Here's how the part is built. I have some questions about the finished solid (model axes, mm). Face numbers are marked on the shaded views. A direction names the side the tool comes from. Round coordinates to 2 decimals unless told otherwise and drop trailing zeros. Order: outer loops, then holes, each group sorted by start corner. A loop starts at its lowest first (then second) coordinate and runs counter-clockwise, first axis right, second up. Notation, with made-up numbers: M -6,-37 L 21,-37 A15 cw 21,-20 Z; hole C 7,-0.75 d4. An arc over 180 degrees is marked long. Use one line per item in the form item = value. Start each with the question number.
```python
from build123d import *
from OCP.BRepFilletAPI import BRepFilletAPI_MakeChamfer

# Parameters (mm, degrees)
SKETCH_1_W               = 126.5
SKETCH_1_H               = 82.5
SKETCH_1_W_2             = 28
SKETCH_1_H_2             = 28
EXTRUDE_1_DEPTH          = 8
SKETCH_2_W               = 126.5
SKETCH_2_H               = 23.75
EXTRUDE_2_DEPTH          = 0.25
CHAMFER_1_SIZE           = 1
CHAMFER_1_SIZE2          = 11.430052303
FILLET_1_R               = 2
FILLET_2_R               = 1
CUT_EXTRUDE_1_DEPTH      = 76.935005103
CUT_EXTRUDE_1_DEPTH_BACK = 76.935005103
SKETCH_3_R               = 2.1
CHAMFER_2_SIZE           = 6
CHAMFER_2_SIZE2          = 3.464101615
CHAMFER_3_SIZE           = 6
CHAMFER_3_SIZE2          = 3.464101615


with BuildPart() as part:
    # Эскиз1 → Бобышка-Вытянуть1 (new body)
    with BuildSketch(Plane(origin=(0, 0, 0), x_dir=(1, 0, 0), z_dir=(0, 1, 0))):
        Rectangle(SKETCH_1_W, SKETCH_1_H)
        Rectangle(SKETCH_1_W_2, SKETCH_1_H_2, mode=Mode.SUBTRACT)
    extrude(amount=EXTRUDE_1_DEPTH)

    # Эскиз2 → Бобышка-Вытянуть2 (add)
    with BuildSketch(Plane(origin=(0, 8, 0), x_dir=(1, 0, 0), z_dir=(0, 1, 0))):
        with Locations((0, 29.375)):
            Rectangle(SKETCH_2_W, SKETCH_2_H)
        with Locations((0, -29.375)):
            Rectangle(SKETCH_2_W, SKETCH_2_H)
    extrude(amount=EXTRUDE_2_DEPTH)

    # Фаска1: one chamfer whose edges measure the first distance from different faces: ONE call of the kernel's chamfer builder (chamfer() names one face for all edges)
    chamfer_1_edges_1 = [part.edges().sort_by_distance(p)[0] for p in [
        (-63.25, 8, 0),
    ]]
    chamfer_1_side_1 = [part.faces().sort_by_distance(p)[0] for p in [
        (-63.25, 4.072906977, 0),
    ]]
    chamfer_1_edges_2 = [part.edges().sort_by_distance(p)[0] for p in [
        (63.25, 8, 0),
    ]]
    chamfer_1_side_2 = [part.faces().sort_by_distance(p)[0] for p in [
        (63.25, 4.072906977, 0),
    ]]
    chamfer_1 = BRepFilletAPI_MakeChamfer(part.part.solid().wrapped)
    for e in chamfer_1_edges_1:
        chamfer_1.Add(CHAMFER_1_SIZE, CHAMFER_1_SIZE2, e.wrapped, chamfer_1_side_1[0].wrapped)  # the first distance lies on this face
    for e in chamfer_1_edges_2:
        chamfer_1.Add(CHAMFER_1_SIZE, CHAMFER_1_SIZE2, e.wrapped, chamfer_1_side_2[0].wrapped)  # the first distance lies on this face
    add(Compound.cast(chamfer_1.Shape()), mode=Mode.REPLACE)

    # Скругление1
    fillet_1_edges = [part.edges().sort_by_distance(p)[0] for p in [
        (63.25, 7, 0),
        (-63.25, 7, 0),
    ]]
    fillet(fillet_1_edges, radius=FILLET_1_R)

    # Скругление2
    fillet_2_edges = [part.edges().sort_by_distance(p)[0] for p in [
        (-14, 8, 0),
        (14, 8, 0),
    ]]
    fillet(fillet_2_edges, radius=FILLET_2_R)

    # Эскиз3 → Вырез-Вытянуть1 (cut, two sides: drawn at the far end of the back side and taken through both)
    with BuildSketch(Plane(origin=(0, 8, 0), x_dir=(1, 0, 0), z_dir=(0, 1, 0)).offset(-CUT_EXTRUDE_1_DEPTH_BACK)):
        with Locations(Location((-40, 30, 0), (0, 0, 270))):
            Circle(SKETCH_3_R)
        with Locations(Location((40, 30, 0), (0, 0, 270))):
            Circle(SKETCH_3_R)
        with Locations(Location((-40, -30, 0), (0, 0, 270))):
            Circle(SKETCH_3_R)
        with Locations(Location((40, -30, 0), (0, 0, 270))):
            Circle(SKETCH_3_R)
    extrude(amount=CUT_EXTRUDE_1_DEPTH + CUT_EXTRUDE_1_DEPTH_BACK, mode=Mode.SUBTRACT)

    # Фаска2: one chamfer whose edges measure the first distance from different faces: ONE call of the kernel's chamfer builder (chamfer() names one face for all edges)
    chamfer_2_edges_1 = [part.edges().sort_by_distance(p)[0] for p in [
        (-14, 0, 0),
    ]]
    chamfer_2_side_1 = [part.faces().sort_by_distance(p)[0] for p in [
        (-14, 3.5, 0),
    ]]
    chamfer_2_edges_2 = [part.edges().sort_by_distance(p)[0] for p in [
        (14, 0, 0),
    ]]
    chamfer_2_side_2 = [part.faces().sort_by_distance(p)[0] for p in [
        (14, 3.5, 0),
    ]]
    chamfer_2 = BRepFilletAPI_MakeChamfer(part.part.solid().wrapped)
    for e in chamfer_2_edges_1:
        chamfer_2.Add(CHAMFER_2_SIZE, CHAMFER_2_SIZE2, e.wrapped, chamfer_2_side_1[0].wrapped)  # the first distance lies on this face
    for e in chamfer_2_edges_2:
        chamfer_2.Add(CHAMFER_2_SIZE, CHAMFER_2_SIZE2, e.wrapped, chamfer_2_side_2[0].wrapped)  # the first distance lies on this face
    add(Compound.cast(chamfer_2.Shape()), mode=Mode.REPLACE)

    # Фаска3: one chamfer whose edges measure the first distance from different faces: ONE call of the kernel's chamfer builder (chamfer() names one face for all edges)
    chamfer_3_edges_1 = [part.edges().sort_by_distance(p)[0] for p in [
        (0, 0, 14),
    ]]
    chamfer_3_side_1 = [part.faces().sort_by_distance(p)[0] for p in [
        (0, 3.837087991, 14),
    ]]
    chamfer_3_edges_2 = [part.edges().sort_by_distance(p)[0] for p in [
        (0, 0, -14),
    ]]
    chamfer_3_side_2 = [part.faces().sort_by_distance(p)[0] for p in [
        (0, 3.837087991, -14),
    ]]
    chamfer_3 = BRepFilletAPI_MakeChamfer(part.part.solid().wrapped)
    for e in chamfer_3_edges_1:
        chamfer_3.Add(CHAMFER_3_SIZE, CHAMFER_3_SIZE2, e.wrapped, chamfer_3_side_1[0].wrapped)  # the first distance lies on this face
    for e in chamfer_3_edges_2:
        chamfer_3.Add(CHAMFER_3_SIZE, CHAMFER_3_SIZE2, e.wrapped, chamfer_3_side_2[0].wrapped)  # the first distance lies on this face
    add(Compound.cast(chamfer_3.Shape()), mode=Mode.REPLACE)


solid = part.part
```
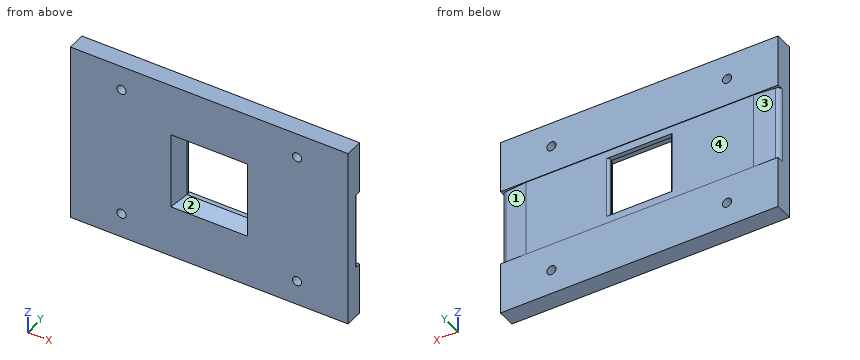
1) If we section it at D-D on z = -30: Write out the boundary of the cut face in (x, y), then the cut area to 3 significant figures.
2) If I drill on line 1 (Z direction, x = -40, y = 3); line 2 (X direction, y = 3, z = -30); line 3 (Z direction, x = -2, y = 6.25), over which ranges is the centre line in solid material (lowest first)?
3) If we section it at A-A on x = 40: Write out the boundary of the cut face in (y, z), then the cut area to 3 significant figures.
4) If we section it at B-B on z = -8: Write out the boundary of the cut face in (x, y), then the cut area to 3 significant figures.
5) If we section it at C-C on x = -7: Write out the boundary of the cut face in (y, z).
6) On a 3-axis mill with a long thin cutter (end or side, diameter ignored), from which of +Z, -Z, +X, -X, +Y, -Y can I reach the whole of each face in a straight line? I mean the marked faces 1, 2, 3 and 4. Say none if no direction works.
7) Will these pins go through, and if not, where does the flat tip stop? pin 1 Ø0.5 at (y, z) = (6.5, -1.5) entering from -X; pin 2 Ø5.5 at (x, z) = (40, 30) entering from -Y; pin 3 Ø1.5 at (x, z) = (50, -2.5) entering from +Y; pin 4 Ø4 at (x, z) = (40, -30) entering from +Y.
Completed:
q1.outline = M -63.25,0 L -42.1,0 L -42.1,8.25 L -63.25,8.25 Z; M -37.9,0 L 37.9,0 L 37.9,8.25 L -37.9,8.25 Z; M 42.1,0 L 63.25,0 L 63.25,8.25 L 42.1,8.25 Z
q1.area = 974 mm²
q2.line_1 = -41.25 to -32.1, -27.9 to 27.9, 32.1 to 41.25
q2.line_2 = -63.25 to -42.1, -37.9 to 37.9, 42.1 to 63.25
q2.line_3 = -41.25 to -14, 14 to 41.25
q3.outline = M 0,-41.25 L 8.25,-41.25 L 8.25,-32.1 L 0,-32.1 Z; M 0,-27.9 L 8.25,-27.9 L 8.25,-17.5 L 8,-17.5 L 8,17.5 L 8.25,17.5 L 8.25,27.9 L 0,27.9 Z; M 0,32.1 L 8.25,32.1 L 8.25,41.25 L 0,41.25 Z
q3.area = 603 mm²
q4.outline = M -63.25,0 L -17.46,0 L -14,6 L -14,7 A1 ccw -15,8 L -51.82,8 L -61.42,7.16 A2 ccw -63.25,5.17 Z; M 14,6 L 17.46,0 L 63.25,0 L 63.25,5.17 A2 ccw 61.42,7.16 L 51.82,8 L 15,8 A1 ccw 14,7 Z
q4.area = 754 mm²
q5.outline = M 0,-41.25 L 8.25,-41.25 L 8.25,-17.5 L 8,-17.5 L 8,-14 L 6,-14 L 0,-17.46 Z; M 0,17.46 L 6,14 L 8,14 L 8,17.5 L 8.25,17.5 L 8.25,41.25 L 0,41.25 Z
q6.face_1 = +X, +Y
q6.face_2 = -Y
q6.face_3 = -X, +Y
q6.face_4 = +X, -X, +Y
q7.pin_1 = -62.93
q7.pin_2 = 0
q7.pin_3 = 8
q7.pin_4 = through
